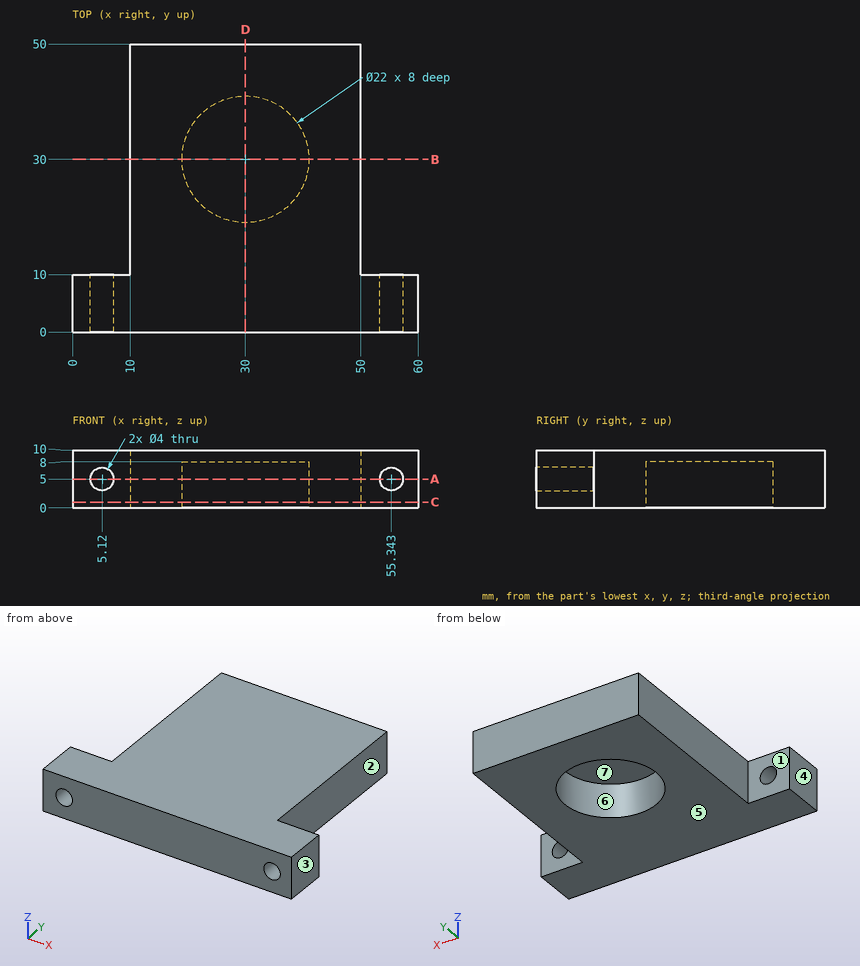
Could you check a few things on this drawing? It's one solid part, dimensions in mm from its lowest x, y, z. A direction names the side the tool comes from. Coordinates: 2 decimals unless noted, no trailing zeros. Loops run counter-clockwise (first coordinate to the right, second up) from the corner with the lowest first, then second, coordinate; pieces in that order, holes last. Notation, with made-up numbers: (70.5, 36.5) - (112.5, 36.5) arc R25 ccw to (112.5, 75.5) - close; hole circle Ø10 at (-0.5, -17). An arc over 180 degrees is marked (long way). Return JSON: item names as keys, results as strings. Group by question number.
Item 1: If we section it at A-A on z = 5: Write out the boundary of the cut face in (x, y).
Item 2: Will these pins go through, and if not, where does the flat tip stop? P1, Ø5, axis at x = 54.5, z = 3, coming from the +Y side; P2, Ø5, axis at y = 26.5, z = 4.5, coming from the -X side; P3, Ø3, axis at y = 20, z = 7, coming from the +X side.
Item 3: If we section it at D-D on x = 30: Write out the boundary of the cut face in (y, z), and give its area (3 significant figures).
Item 4: On a 3-axis mill with a long thin cutter (end or side, diameter ignored), from which of +Z, -Z, +X, -X, +Y, -Y can I reach the whole of each face in a straight line? I mean the marked faces 1, 2 and 3. Say none if no direction works.
Item 5: We'd pull the mould along X, two halves only. Please class the marked faces 4, 5, 6 and 7: +X half, -X half, draft (parallel to the pull), parting line (faces both ways), or undercut.
Item 6: If we section it at B-B on y = 30: Write out the boundary of the cut face in (x, z), and give its area (3 significant figures).
Item 7: If we section it at C-C on z = 1: Write out the boundary of the cut face in (x, y).
Item 8: I need wall thicknesses on line 1 (X direction, y = 6.75, z = 5); line 2 (Y direction, x = 30, z = 3.5); line 3 (X direction, y = 3.5, z = 5.25) (1 decimal). Which ranges of each line are inside material? Lowest first, please. Write a range as from..to.
Calculated:
{
 "1": {"outline": "(0, 0) - (3.12, 0) - (3.12, 10) - (0, 10) - close; (7.12, 0) - (53.34, 0) - (53.34, 10) - (50, 10) - (50, 50) - (10, 50) - (10, 10) - (7.12, 10) - close; (57.34, 0) - (60, 0) - (60, 10) - (57.34, 10) - close; hole circle Ø22 at (30, 30)"},
 "2": {"P1": "stops at y = 10", "P2": "stops at x = 10", "P3": "stops at x = 50"},
 "3": {"outline": "(0, 0) - (19, 0) - (19, 8) - (41, 8) - (41, 0) - (50, 0) - (50, 10) - (0, 10) - close", "area": "324 mm^2"},
 "4": {"face 1": "+Z, -Z, -X, +Y", "face 2": "+Z, -Z, +X, +Y", "face 3": "+Z, -Z, +X, +Y, -Y"},
 "5": {"face 4": "-X half", "face 5": "draft", "face 6": "undercut", "face 7": "undercut"},
 "6": {"outline": "(10, 0) - (19, 0) - (19, 8) - (41, 8) - (41, 0) - (50, 0) - (50, 10) - (10, 10) - close", "area": "224 mm^2"},
 "7": {"outline": "(0, 0) - (60, 0) - (60, 10) - (50, 10) - (50, 50) - (10, 50) - (10, 10) - (0, 10) - close; hole circle Ø22 at (30, 30)"},
 "8": {"line 1": "x = 0..3.12, 7.12..53.34, 57.34..60", "line 2": "y = 0..19, 41..50", "line 3": "x = 0..3.1, 7.1..53.4, 57.3..60"}
}
